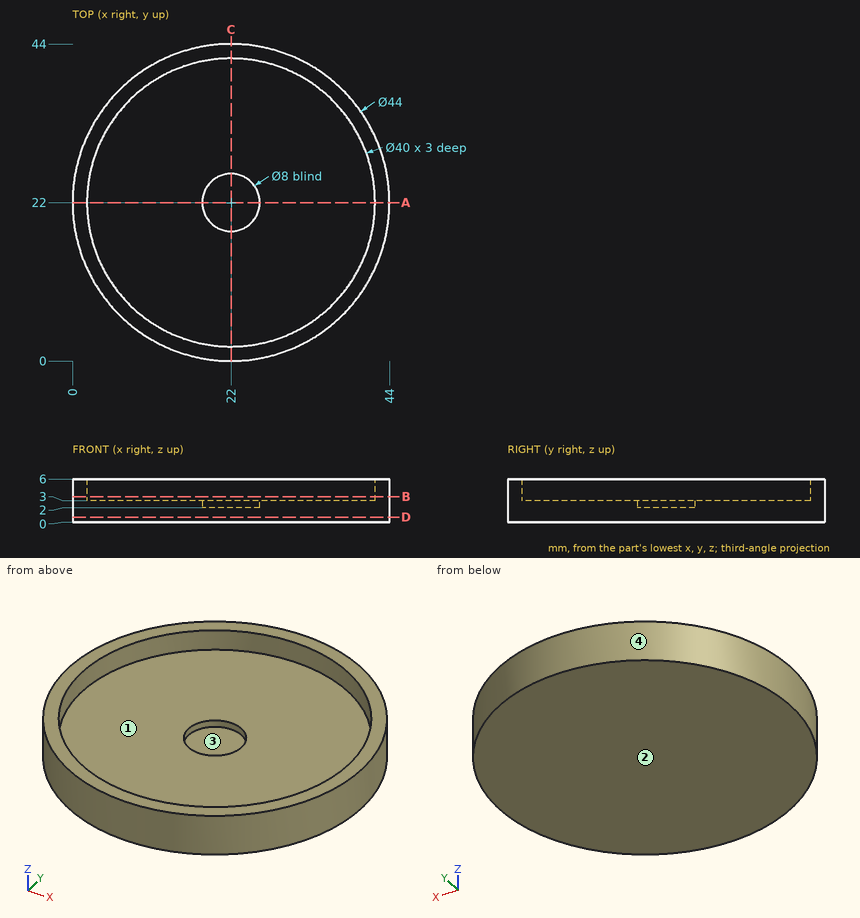
Design review of the part shown in the three views and the two pictorial views. Dimensions are in mm from the part's minimum x, y and z. Coordinates: 2 decimals unless noted, no trailing zeros. Write each loop counter-clockwise with the first axis right and the second up, starting at its lowest first coordinate (ties: lowest second). Pieces come first, ordered by that corner, then holes.
(1) The part is to be moulded in two halves that separate along X. For the marked faces 1, 2, 3 and 4, say which applies: +X half, -X half, draft (parallel to the pull), parting line (faces both ways), or undercut.
(2) Add section B-B on z = 3.55. Give the boundary of the cut face in (x, y), then the cut area to 3 significant figures.
(3) For pin 1 Ø3 at (x, z) = (31.5, 1) entering from -Y; pin 2 Ø12 at (x, y) = (8, 23) entering from -Z; pin 3 Ø1 at (x, y) = (12.5, 37) entering from +Z; pin 4 Ø2 at (y, z) = (7, 4.5) entering from +X, all flat-tipped, find the tip position at first contact; note any pin that passes through.
(4) Add section A-A on y = 22. Give the boundary of the cut face in (x, z), then the cut area to 3 significant figures.
(5) Wall thickness on probe 1 along Y at (x, z) = (22, 5.3); probe 2 along Y at (x, z) = (22, 2.2); probe 3 along Z at (x, y) = (13, 30.5): over which ranges is each line inside the solid? List them lowest first.
(6) Add section D-D on z = 0.7. Give the boundary of the cut face in (x, y).
Answer sheet:
1. face 1: undercut
1. face 2: draft
1. face 3: undercut
1. face 4: parting line
2. outline: circle Ø44 at (22, 22); hole circle Ø40 at (22, 22)
2. area: 264 mm2
3. pin 1: stops at y = 1.51
3. pin 2: stops at z = 0
3. pin 3: stops at z = 3
3. pin 4: stops at x = 38.97
4. outline: (0, 0) - (44, 0) - (44, 6) - (42, 6) - (42, 3) - (26, 3) - (26, 2) - (18, 2) - (18, 3) - (2, 3) - (2, 6) - (0, 6) - close
4. area: 136 mm2
5. probe 1: y = 0 to 2, 42 to 44
5. probe 2: y = 0 to 18, 26 to 44
5. probe 3: z = 0 to 3
6. outline: circle Ø44 at (22, 22)
